Design review of the part shown in the three views and the two pictorial views. Dimensions are in mm from the part's minimum x, y and z. A direction names the side the tool comes from. Coordinates: 2 decimals unless noted, no trailing zeros. Write each loop counter-clockwise with the first axis right and the second up, starting at its lowest first coordinate (ties: lowest second). Pieces come first, ordered by that corner, then holes. Notation, with made-up numbers: (85, 1) - (95, 1) arc R5 cw to (95, 5) - close; hole circle Ø1 at (86, -34). An arc over 180 degrees is marked (long way). Return JSON: item names as keys, results as strings. Group by question number.
(1) Tool access review of the marked faces 1 and 2: name each direction out of +Z, -Z, +X, -X, +Y, -Y from which nothing blocks a thin tool from reaching the whole face with its end or side.
(2) Draft analysis for pull direction Z (two halves, no side actions). For the marked faces 3 and 4, state which applies: released by +Z, released by -Z, zero draft, split by the parting line, or undercut.
(3) For pin 1 Ø15 at (x, z) = (125.5, 123.5) entering from +Y; pin 2 Ø15 at (x, y) = (171, 31.5) entering from +Z; pin 3 Ø25 at (y, z) = (21, 130.5) entering from +X, all flat-tipped, find the tip position at first contact; note any pin that passes through.
(4) To check wall thickness, follow L1, parallel to X at y = 84, z = 193.5; L2, parallel to Z at x = 215, y = 24.5; L3, parallel to Y at x = 284, z = 490. State the ranges of each line that lie inside material, in increasing order. Write a range as from..to.
(5) We need section C-C on z = 141.5. State the section outline as (x, y) points, then the cut area to 3 significant figures.
(6) We need section B-B on x = 335. State the section outline as (y, z) points.
(7) We need section A-A on y = 38. State the section outline as (x, z) points.
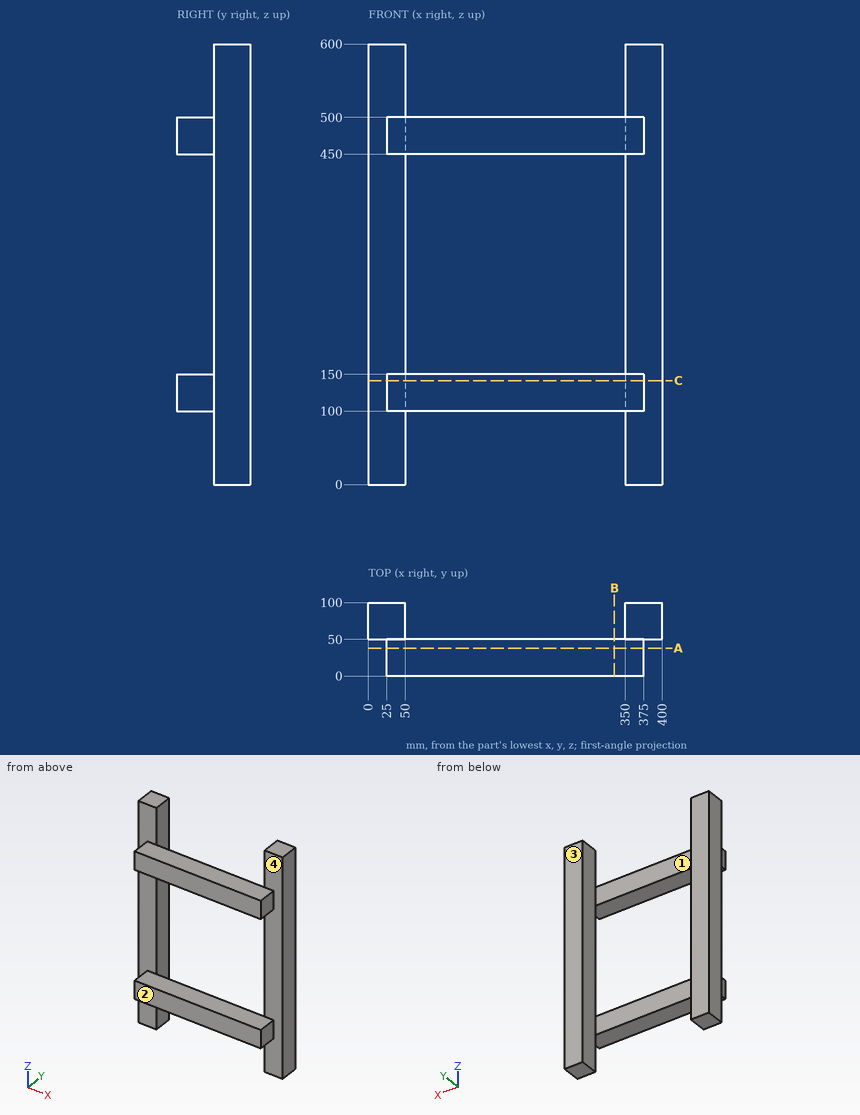
Ans:
{
 "1": {"face 1": "+Z, -Z, +Y", "face 2": "+Z, -Z, +X, -X, -Y"},
 "2": {"face 3": "zero draft", "face 4": "undercut"},
 "3": {"pin 1": "y = 50", "pin 2": "z = 500", "pin 3": "x = 375"},
 "4": {"L1": "0..50, 350..400", "L2": "100..150, 450..500", "L3": "0..50"},
 "5": {"outline": "(0, 50) - (25, 50) - (25, 0) - (375, 0) - (375, 50) - (400, 50) - (400, 100) - (350, 100) - (350, 50) - (50, 50) - (50, 100) - (0, 100) - close", "area": "22,500 mm²"},
 "6": {"outline": "(0, 100) - (50, 100) - (50, 150) - (0, 150) - close; (0, 450) - (50, 450) - (50, 500) - (0, 500) - close"},
 "7": {"outline": "(25, 100) - (375, 100) - (375, 150) - (25, 150) - close; (25, 450) - (375, 450) - (375, 500) - (25, 500) - close"}
}
